from build123d import *

# Parameters (mm, degrees)
SKETCH2_W           = 25.4
SKETCH2_H           = 25.4
SKETCH6_W           = 25.4
SKETCH6_H           = 25.4
SKETCH7_W           = 25.4
SKETCH7_H           = 100
BOSS_EXTRUDE1_DEPTH = 974.6
SKETCH8_W           = 150
SKETCH8_H           = 25.4
BOSS_EXTRUDE2_DEPTH = 324.6
SKETCH14_R          = 26
CUT_EXTRUDE1_DEPTH  = 1115


with BuildPart() as part:
    # Sweep4: sweep along a path in Sketch1
    with BuildLine(Plane(origin=(0, 0, 0), x_dir=(1, 0, 0), z_dir=(0, 1, 0))) as sweep4_path:
        Line((-350, -500), (350, -500))
        Line((350, -500), (350, 500))
        Line((350, 500), (-350, 500))
        Line((-350, 500), (-350, -500))
    # Sketch2 → Sweep4 (sweep)
    with BuildSketch(Plane(origin=(0, 0, 0), x_dir=(0, 0, -1), z_dir=(1, 0, 0))):
        with Locations((500, 0)):
            Rectangle(SKETCH2_W, SKETCH2_H)
    sweep(path=sweep4_path.line, transition=Transition.RIGHT)

    # Sweep5: sweep along a path in Sketch4
    with BuildLine(Plane(origin=(0, 0, 0), x_dir=(0, 0, -1), z_dir=(1, 0, 0))) as sweep5_path:
        Line((-500, 0), (-500, 1000))
        Line((-500, 1000), (500, 1000))
        Line((500, 1000), (500, 0))
        Line((500, 0), (-500, 0))
    # Sketch6 → Sweep5 (sweep)
    with BuildSketch(Plane(origin=(0, 12.7, 0), x_dir=(1, 0, 0), z_dir=(0, 1, 0))):
        with Locations((0, 500)):
            Rectangle(SKETCH6_W, SKETCH6_H)
    sweep(path=sweep5_path.line, transition=Transition.RIGHT)

    # Sketch7 → Boss-Extrude1 (add)
    with BuildSketch(Plane(origin=(0, 12.7, 0), x_dir=(1, 0, 0), z_dir=(0, 1, 0))):
        Polygon((-12.7, -25), (-12.7, -50), (12.7, -50), (12.7, -25), (12.7, 25), (12.7, 50), (-12.7, 50), (-12.7, 25), align=None)
        with Locations((0, -270.176844268)):
            Rectangle(SKETCH7_W, SKETCH7_H)
        with Locations((0, 300)):
            Rectangle(SKETCH7_W, SKETCH7_H)
    extrude(amount=BOSS_EXTRUDE1_DEPTH)

    # Sketch8 → Boss-Extrude2 (add)
    with BuildSketch(Plane.ZY.offset(12.7)):
        with Locations((-300, 0)):
            Rectangle(SKETCH8_W, SKETCH8_H)
        Rectangle(SKETCH8_W, SKETCH8_H)
        with Locations((300, 0)):
            Rectangle(SKETCH8_W, SKETCH8_H)
    extrude(amount=BOSS_EXTRUDE2_DEPTH)

    # Sketch14 → Cut-Extrude1 (cut)
    with BuildSketch(Plane(origin=(12.7, 0, 0), x_dir=(0, 0, -1), z_dir=(1, 0, 0))):
        with Locations((-270.176844268, 762.7)):
            Circle(SKETCH14_R)
        with Locations((-0.176844268, 762.7)):
            Circle(SKETCH14_R)
        with Locations((299.823155732, 762.7)):
            Circle(SKETCH14_R)
        with Locations((-270.176844268, 262.7)):
            Circle(SKETCH14_R)
        with Locations((-0.176844268, 262.7)):
            Circle(SKETCH14_R)
        with Locations((299.823155732, 262.7)):
            Circle(SKETCH14_R)
    extrude(amount=-CUT_EXTRUDE1_DEPTH, mode=Mode.SUBTRACT)


solid = part.part
The listing builds one solid part. Answer for the finished solid, in the listing's coordinates (mm). A direction names the side the tool comes from. Give positions to 0.01 mm unless a question says otherwise; leave off trailing zeros. Write each loop counter-clockwise with the first axis right and the second up, starting at its lowest first coordinate (ties: lowest second). Pieces come first, ordered by that corner, then holes.
Item 1: Which of the six approach directions +Z, -Z, +X, -X, +Y, -Y give full straight-line access (tool end or side, diameter ignored) to faces 1 (the flat face through (0, 987.3, -420)), 2 (the flat face through (-173, 0, -75)), 3 (the flat face through (-133, -12.7, -2))?
Item 2: Section D-D, the plane z = -178.5 is taken. Write down the section's boundary in (x, y), plus the area to 3 significant figures.
Item 3: A flat-ended cylindrical pin translates along its axis: P1, Ø6, axis at y = 231.5, z = 22.5, coming from the +X side. Find the tip coordinate at first contact, or state that the pin passes through.
Item 4: Find the intervals of material crossed by line 1 along Z through (x, y) = (5, 554.5); line 2 along Y through (x, z) = (-151, 364), in increasing order.
Item 5: Section B-B, the plane x = -117 is taken. Write down the section's boundary in (y, z).
Item 6: Section A-A, the plane z = 334.5 is taken. Write down the section's boundary in (x, y), plus the area to 3 significant figures.
Item 7: Section C-C, the plane y = 599.5 is taken. Write down the section's boundary in (x, z).
Item 8: Determine the mould class of faces 4 (the flat face through (337.3, 0, -7)), 5 (the flat face through (-173, 0, 225)), 6 (the flat face through (-2, 270, -512.7)) for opening direction X: released by +X, released by -X, zero draft, split by the parting line, or undercut.
Completed:
1. face 1: +X, -X
1. face 2: +Y, -Y
1. face 3: +Z, -Z, +X, -X, -Y
2. outline: (-362.7, -12.7) - (-337.3, -12.7) - (-337.3, 12.7) - (-362.7, 12.7) - close; (-12.7, -12.7) - (12.7, -12.7) - (12.7, 12.7) - (-12.7, 12.7) - close; (-12.7, 987.3) - (12.7, 987.3) - (12.7, 1012.7) - (-12.7, 1012.7) - close; (337.3, -12.7) - (362.7, -12.7) - (362.7, 12.7) - (337.3, 12.7) - close
2. area: 2,580 mm2
3. P1: stops at x = 12.7
4. line 1: z = -512.7 to -487.3, -350 to -250, -50 to 50, 220.18 to 320.18, 487.3 to 512.7
4. line 2: y = -12.7 to 12.7
5. outline: (-12.7, -512.7) - (12.7, -512.7) - (12.7, -487.3) - (-12.7, -487.3) - close; (-12.7, -375) - (12.7, -375) - (12.7, -225) - (-12.7, -225) - close; (-12.7, -75) - (12.7, -75) - (12.7, 75) - (-12.7, 75) - close; (-12.7, 225) - (12.7, 225) - (12.7, 375) - (-12.7, 375) - close; (-12.7, 487.3) - (12.7, 487.3) - (12.7, 512.7) - (-12.7, 512.7) - close
6. outline: (-362.7, -12.7) - (12.7, -12.7) - (12.7, 12.7) - (-362.7, 12.7) - close; (-12.7, 987.3) - (12.7, 987.3) - (12.7, 1012.7) - (-12.7, 1012.7) - close; (337.3, -12.7) - (362.7, -12.7) - (362.7, 12.7) - (337.3, 12.7) - close
6. area: 10,800 mm2
7. outline: (-12.7, -512.7) - (12.7, -512.7) - (12.7, -487.3) - (-12.7, -487.3) - close; (-12.7, -350) - (12.7, -350) - (12.7, -250) - (-12.7, -250) - close; (-12.7, -50) - (12.7, -50) - (12.7, 50) - (-12.7, 50) - close; (-12.7, 220.18) - (12.7, 220.18) - (12.7, 320.18) - (-12.7, 320.18) - close; (-12.7, 487.3) - (12.7, 487.3) - (12.7, 512.7) - (-12.7, 512.7) - close
8. face 4: undercut
8. face 5: undercut
8. face 6: zero draft
